Source: CAD feature listing. Evaluate the final solid. Frame: model axes, mm. A direction names the side the tool comes from. Coordinates: 2 decimals unless noted, no trailing zeros. Write each loop counter-clockwise with the first axis right and the second up, starting at its lowest first coordinate (ties: lowest second). Pieces come first, ordered by that corner, then holes. Notation, with made-up numbers: M 12,24 L 62,24 A29 cw 62,56 Z; hole C 74.5,-26 d9. An arc over 180 degrees is marked long. Answer as CSV lines item,"result". Start each with the question number.
1. Mould query, pull axis X, two halves, no side actions, for faces 1 (the face through (7, 19, 49)), 2 (the face through (0, 0, 100)), 3 (the face through (-0.89, -22.482, 50.314)). Classes: pulls with the +X half, pulls with the -X half, needs draft (parallel to the pull), parting line crosses it, or undercut.
2. Section B-B on x = 0. Return the cut outline in (y, z).
3. Contact query for flat-ended pins moving along their axis: pin 1 Ø4 at (y, z) = (0.5, 89) entering from +X; pin 2 Ø1.2 at (y, z) = (19, 65) entering from +X; pin 3 Ø8 at (y, z) = (-8, 17) entering from -X; pin 4 Ø1.5 at (y, z) = (10, 22.5) entering from -X. Output: stop coordinate, or through.
4. Line query: probe 1 along X at (y, z) = (-1.5, 36); probe 2 along X at (y, z) = (-15, 19); probe 3 along Y at (x, z) = (16.5, 77.5). Output: solid intervals per line, ascending. Write a range as [from, to].
5. Reachability of faces 4 (the face through (0, 0, 0)), 5 (the face through (-7, 19, 49)) from +Z, -Z, +X, -X, +Y, -Y: full face, straight path, thin tool, end or side. Return the list, or none.
6. Section A-A on z = 52. Return the cut outline in (x, y), plus the area to 3 significant figures.
```python
from build123d import *

# Parameters (mm, degrees)
SKETCH1_R           = 22.5
BOSS_EXTRUDE3_DEPTH = 100
SKETCH5_W           = 14
SKETCH5_H           = 7.800985848
CUT_EXTRUDE2_DEPTH  = 100
FILLET1_R           = 2


with BuildPart() as part:
    # Sketch1 → Boss-Extrude3 (new body)
    with BuildSketch(Plane.XY):
        Circle(SKETCH1_R)
    extrude(amount=BOSS_EXTRUDE3_DEPTH)

    # Sketch5 → Cut-Extrude2 (cut)
    with BuildSketch(Plane(origin=(0, 0, 0), x_dir=(-1, 0, 0), z_dir=(0, 0, -1))):
        with Locations((0, 21.400492924)):
            Rectangle(SKETCH5_W, SKETCH5_H)
    extrude(amount=-CUT_EXTRUDE2_DEPTH, mode=Mode.SUBTRACT)

    # Fillet1
    fillet1_edges = [part.edges().sort_by_distance(p)[0] for p in [
        (0, -22.5, 0),
    ]]
    fillet(fillet1_edges, radius=FILLET1_R)


solid = part.part
```
Values:
1,face 1,"undercut"
1,face 2,"needs draft"
1,face 3,"parting line crosses it"
2,outline,"M -22.5,2 A2 ccw -20.5,0 L 17.5,0 L 17.5,100 L -22.5,100 Z"
3,pin 1,"x = 22.5"
3,pin 2,"x = 12.95"
3,pin 3,"x = -22.14"
3,pin 4,"x = -20.51"
4,probe 1,"[-22.45, 22.45]"
4,probe 2,"[-16.77, 16.77]"
4,probe 3,"[-15.3, 15.3]"
5,face 4,"-Z, +X, -X, +Y, -Y"
5,face 5,"+Z, -Z, +Y"
6,outline,"M -7,17.5 L -7,21.38 A22.5 ccw long 7,21.38 L 7,17.5 Z"
6,area,"1,530 mm²"
